Here's how the part is built. I have some questions about the finished solid (model axes, mm). Face numbers are marked on the shaded views. A direction names the side the tool comes from. Round coordinates to 2 decimals unless told otherwise and drop trailing zeros. Write each loop counter-clockwise with the first axis right and the second up, starting at its lowest first coordinate (ties: lowest second). Pieces come first, ordered by that corner, then holes. Notation, with made-up numbers: (-12.5, 57.25) -> (43.5, 57.25) arc R30 cw to (43.5, 83.25) -> close; hole circle Ø9 at (-2, 56.25). An arc over 180 degrees is marked (long way). Put each result on its own line as item: value. Start each with the question number.
1. Suppose I cut it at A-A (y = 0). Please give me the cut outline in (x, z) (3 decimals), then the cut area to 3 significant figures.
2. Suppose I cut it at C-C (z = 41). Please give me the cut outline in (x, y) (3 decimals).
3. Which directions (+Z, -Z, +X, -X, +Y, -Y) give clear straight access to the entire face, cutting with the end or side of a thin tool? Please do the marked faces 1 and 2.
4. For pin 1 (1 mm diameter, centred on y = 5.5, z = 58.5, fed in from -X); pin 2 (3.5 mm diameter, centred on x = -15, y = 0.5, fed in from +Z); pin 3 (0.9 mm diameter, centred on x = 8, y = -12.5, fed in from +Z), each with a flat end and sliding along its axis, tell me the tip position at first contact or that it passes through.
5. Suppose I cut it at D-D (x = 15). Please give me the cut outline in (y, z), then the cut area to 3 significant figures.
6. I need wall thicknesses on probe 1 along Y at (x, z) = (-6.5, 52); probe 2 along Z at (x, y) = (-4, 5); probe 3 along X at (y, z) = (-13.5, 47.5). Which ranges of each line are inside material? Lowest first, please. Write a range as from..to.
7. Suppose I cut it at B-B (x = -8). Please give me the cut outline in (y, z).
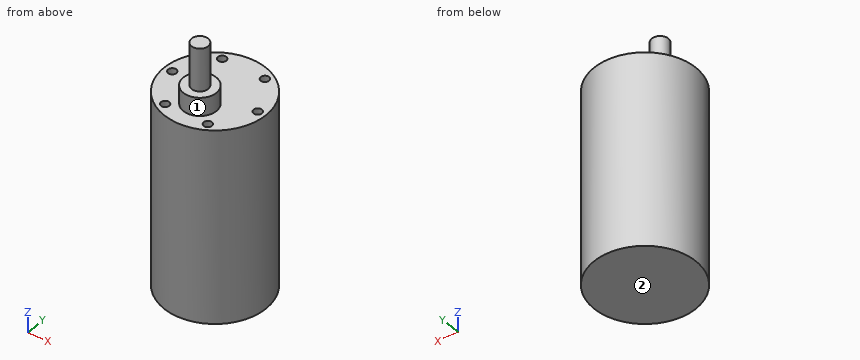
```python
from build123d import *

# Parameters (mm, degrees)
SKETCH1_R           = 18.415
BOSS_EXTRUDE1_DEPTH = 70.104
SKETCH2_R           = 5.969
BOSS_EXTRUDE2_DEPTH = 6.604
SKETCH3_R           = 3
BOSS_EXTRUDE3_DEPTH = 15.494
SKETCH4_R           = 1.5
CUT_EXTRUDE1_DEPTH  = 25.4


with BuildPart() as part:
    # Sketch1 → Boss-Extrude1 (new body)
    with BuildSketch(Plane.XY):
        Circle(SKETCH1_R)
    extrude(amount=BOSS_EXTRUDE1_DEPTH)

    # Sketch2 → Boss-Extrude2 (add)
    with BuildSketch(Plane.XY.offset(70.104)):
        with Locations(Location((0, -7.112, 0), (0, 0, 180))):
            Circle(SKETCH2_R)
    extrude(amount=BOSS_EXTRUDE2_DEPTH)

    # Sketch3 → Boss-Extrude3 (add)
    with BuildSketch(Plane.XY.offset(76.708)):
        with Locations((0, -7.112)):
            Circle(SKETCH3_R)
    extrude(amount=BOSS_EXTRUDE3_DEPTH)

    # Sketch4 → Cut-Extrude1 (cut)
    with BuildSketch(Plane.XY.offset(70.104)):
        with Locations((-15.494, 0)):
            Circle(SKETCH4_R)
        with Locations((15.494, 0)):
            Circle(SKETCH4_R)
        with Locations((7.747, 13.418197606)):
            Circle(SKETCH4_R)
        with Locations((-7.747, 13.418197606)):
            Circle(SKETCH4_R)
        with Locations((-7.747, -13.418197606)):
            Circle(SKETCH4_R)
        with Locations((7.747, -13.418197606)):
            Circle(SKETCH4_R)
    extrude(amount=-CUT_EXTRUDE1_DEPTH, mode=Mode.SUBTRACT)


solid = part.part
```
Verdict:
1. outline: (-18.415, 0) -> (18.415, 0) -> (18.415, 70.104) -> (16.994, 70.104) -> (16.994, 44.704) -> (13.994, 44.704) -> (13.994, 70.104) -> (-13.994, 70.104) -> (-13.994, 44.704) -> (-16.994, 44.704) -> (-16.994, 70.104) -> (-18.415, 70.104) -> close
1. area: 2,430 mm^2
2. outline: circle Ø36.83 at (0, 0)
3. face 1: +Z
3. face 2: -Z, +X, -X, +Y, -Y
4. pin 1: stops at x = -17.72
4. pin 2: stops at z = 70.1
4. pin 3: stops at z = 44.7
5. outline: (-10.68, 0) -> (10.68, 0) -> (10.68, 70.1) -> (1.42, 70.1) -> (1.42, 44.7) -> (-1.42, 44.7) -> (-1.42, 70.1) -> (-10.68, 70.1) -> close
5. area: 1,430 mm^2
6. probe 1: y = -17.23..-14.25, -12.58..12.58, 14.25..17.23
6. probe 2: z = 0..70.1
6. probe 3: x = -12.52..-9.24, -6.25..6.25, 9.24..12.52
7. outline: (-16.59, 0) -> (16.59, 0) -> (16.59, 70.1) -> (14.9, 70.1) -> (14.9, 44.7) -> (11.94, 44.7) -> (11.94, 70.1) -> (-11.94, 70.1) -> (-11.94, 44.7) -> (-14.9, 44.7) -> (-14.9, 70.1) -> (-16.59, 70.1) -> close
